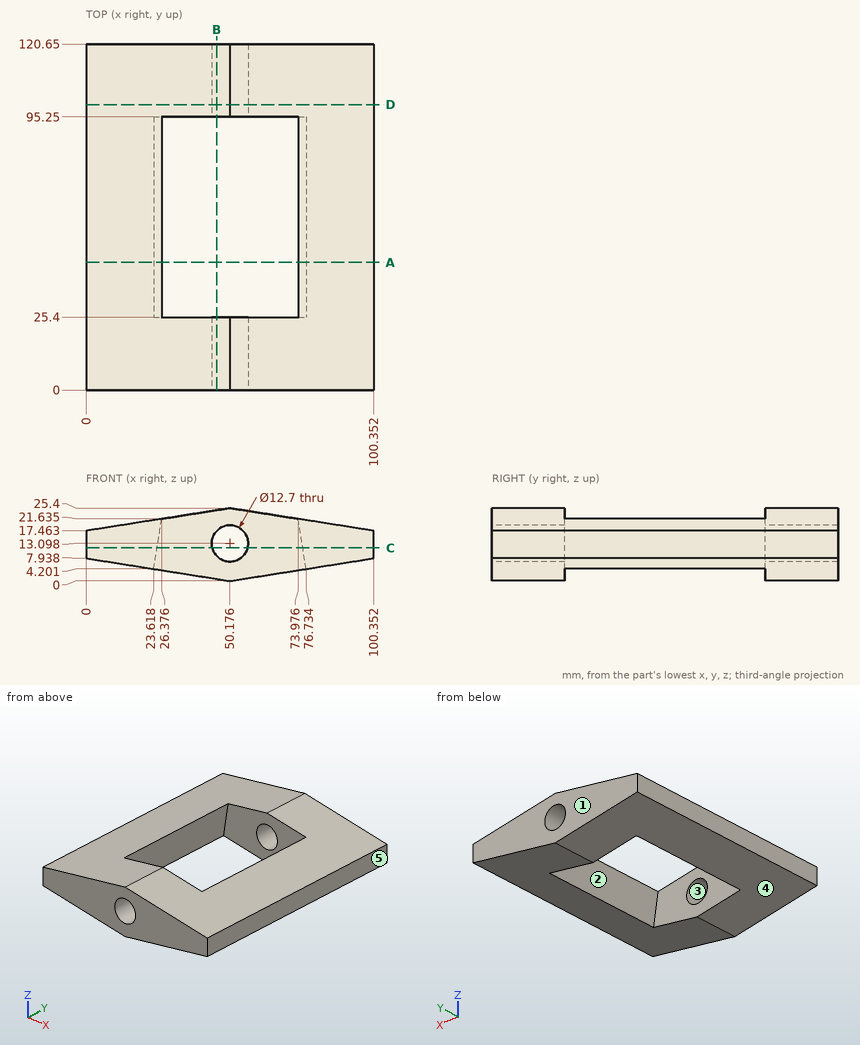
Could you check a few things on this drawing? It's one solid part, dimensions in mm from its lowest x, y, z. A direction names the side the tool comes from. Give positions to 0.01 mm unless a question says otherwise; leave off trailing zeros. Write each loop counter-clockwise with the first axis right and the second up, starting at its lowest first coordinate (ties: lowest second). Pieces come first, ordered by that corner, then holes. Notation, with made-up numbers: M 21.25,-29 L 67.25,-29 A24 cw 67.25,-4 Z; hole C 11,-13.75 d2. An arc over 180 degrees is marked long. Put each result on its own line as item: value. Start each with the question number.
Item 1: I need wall thicknesses on L1, parallel to Y at x = 62, z = 18.25; L2, parallel to X at y = 105.5, z = 15.75 (1 decimal); L3, parallel to X at y = 87.5, z = 12. Which ranges of each line are inside material? Lowest first, please. Write a range as from..to.
Item 2: Thinking about a two-plate mould opening in X: for the marked faces 3, 4 and 5, which applies, +X half, -X half, draft (parallel to the pull), parting line (faces both ways), or undercut?
Item 3: If we section it at B-B, the plane x = 45.5: Write out the boundary of the cut face in (y, z).
Item 4: On a 3-axis mill with a long thin cutter (end or side, diameter ignored), from which of +Z, -Z, +X, -X, +Y, -Y can I reach the whole of each face in a straight line? I mean the marked faces 1 and 2. Say none if no direction works.
Item 5: If we section it at C-C, the plane z = 11.5: Write out the boundary of the cut face in (x, y).
Item 6: If we section it at A-A, the plane y = 44.5: Write out the boundary of the cut face in (x, z) (1 decimal), then the cut area to 3 significant figures.
Item 7: If we section it at D-D, the plane y = 99.5: Write out the boundary of the cut face in (x, z).
Values:
1. L1: 0..25.4, 95.25..120.65
1. L2: 0..44.4, 55.9..100.4
1. L3: 0..24.85, 75.5..100.35
2. face 3: undercut
2. face 4: -X half
2. face 5: +X half
3. outline: M 0,0.74 L 25.4,0.74 L 25.4,8.8 L 0,8.8 Z; M 0,17.39 L 25.4,17.39 L 25.4,24.66 L 0,24.66 Z; M 95.25,0.74 L 120.65,0.74 L 120.65,8.8 L 95.25,8.8 Z; M 95.25,17.39 L 120.65,17.39 L 120.65,24.66 L 95.25,24.66 Z
4. face 1: +Z, -Z, +X, -X, +Y
4. face 2: -Z
5. outline: M 0,0 L 44.03,0 L 44.03,25.4 L 24.77,25.4 L 24.77,95.25 L 44.03,95.25 L 44.03,120.65 L 0,120.65 Z; M 56.32,0 L 100.35,0 L 100.35,120.65 L 56.32,120.65 L 56.32,95.25 L 75.58,95.25 L 75.58,25.4 L 56.32,25.4 Z
6. outline: M 0,7.9 L 23.6,4.2 L 26.4,21.6 L 0,17.5 Z; M 74,21.6 L 76.7,4.2 L 100.4,7.9 L 100.4,17.5 Z
6. area: 673 mm²
7. outline: M 0,7.94 L 50.18,0 L 100.35,7.94 L 100.35,17.46 L 50.18,25.4 L 0,17.46 Z; hole C 50.18,13.1 d12.7
